The drawing under review shows one solid part. Ordinate dimensions are in mm from its lowest x, y, z. A direction names the side the tool comes from. Round coordinates to 2 decimals unless told otherwise and drop trailing zeros. Write each loop counter-clockwise with the first axis right and the second up, starting at its lowest first coordinate (ties: lowest second). Pieces come first, ordered by that corner, then holes. Notation, with made-up numbers: M 10,21.5 L 19,21.5 A21 cw 19,43.5 Z; hole C 85.25,-32 d5. An arc over 180 degrees is marked long. Write item = value, one per line. Start each with the question number.
Item 1: The part is to be moulded in two halves that separate along X. For the marked faces 1, 2, 3 and 4, say which applies: +X half, -X half, draft (parallel to the pull), parting line (faces both ways), or undercut.
Item 2: Tool access review of the marked faces 5 and 6: name each direction out of +Z, -Z, +X, -X, +Y, -Y from which nothing blocks a thin tool from reaching the whole face with its end or side.
Item 3: Take a section at B-B, the plane z = 3.2. Give the boundary of the cut face in (x, y).
Item 4: For pin 1 Ø5 at (x, y) = (20.5, 6) entering from +Z; pin 2 Ø1.3 at (x, y) = (43.5, 1.75) entering from -Z; pin 3 Ø1.7 at (x, y) = (42.5, 9.5) entering from +Z, all flat-tipped, find the tip position at first contact; note any pin that passes through.
Item 5: Take a section at C-C, the plane x = 44. Give the boundary of the cut face in (y, z).
Item 6: Take a section at A-A, the plane y = 1.75. Give the boundary of the cut face in (x, z), plus the area to 3 significant figures.
Item 7: Take a section at D-D, the plane y = 7.25. Give the boundary of the cut face in (x, z), plus the area to 3 significant figures.
Item 8: To check wall thickness, follow line 1 along Y through (x, z) = (43.5, 0.85); line 2 along X through (y, z) = (7.25, 3); line 3 along X through (y, z) = (14.5, 1). State the ranges of each line that lie inside material, in increasing order.
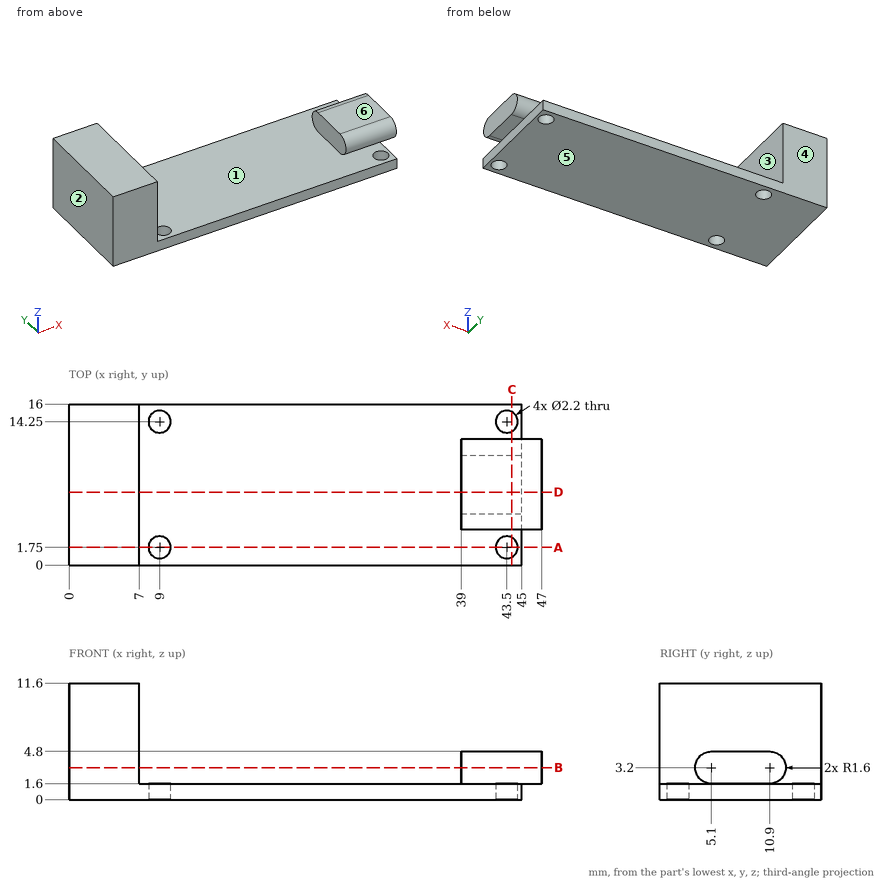
Response values:
q1.face_1 = undercut
q1.face_2 = -X half
q1.face_3 = undercut
q1.face_4 = draft
q2.face_5 = -Z, +X, -X, +Y, -Y
q2.face_6 = +Z, +X, +Y, -Y
q3.outline = M 0,0 L 7,0 L 7,16 L 0,16 Z; M 39,3.5 L 47,3.5 L 47,12.5 L 39,12.5 Z
q4.pin_1 = 1.6
q4.pin_2 = through
q4.pin_3 = 4.8
q5.outline = M 0,0 L 0.77,0 L 0.77,1.6 L 0,1.6 Z; M 2.73,0 L 13.27,0 L 13.27,1.6 L 10.9,1.6 A1.6 ccw 10.9,4.8 L 5.1,4.8 A1.6 ccw 5.1,1.6 L 2.73,1.6 Z; M 15.23,0 L 16,0 L 16,1.6 L 15.23,1.6 Z
q6.outline = M 0,0 L 7.9,0 L 7.9,1.6 L 7,1.6 L 7,11.6 L 0,11.6 Z; M 10.1,0 L 42.4,0 L 42.4,1.6 L 10.1,1.6 Z; M 44.6,0 L 45,0 L 45,1.6 L 44.6,1.6 Z
q6.area = 135 mm2
q7.outline = M 0,0 L 45,0 L 45,1.6 L 47,1.6 L 47,4.8 L 39,4.8 L 39,1.6 L 7,1.6 L 7,11.6 L 0,11.6 Z
q7.area = 168 mm2
q8.line_1 = 0 to 0.65, 2.85 to 13.15, 15.35 to 16
q8.line_2 = 0 to 7, 39 to 47
q8.line_3 = 0 to 7.93, 10.07 to 42.43, 44.57 to 45
